```python
from build123d import *

# Parameters (mm, degrees)
F1_DEPTH    = 2500
F2_T        = 5
F2_T3_DEPTH = 2510
F4_DEPTH    = 2


# Not quite as in the source:
# - a shell that OpenCascade refuses in one call is made with other operations: the cavity is built on its own and cut out


with BuildPart() as f1:
    # F0 (on Top) → F1 (new body)
    with BuildSketch(Plane.XY):
        with BuildLine():
            Line((243.3531384634, 9.5), (16.4544826719, 140.5))
            ThreePointArc((16.4544826719, 140.5), (10.418948766, 139.705406887), (9.624355653, 133.6698729811))
            Line((9.624355653, 133.6698729811), (10.874355653, 131.5048094716))
            Line((10.874355653, 131.5048094716), (10.5801270189, 131.3349364905))
            Line((10.5801270189, 131.3349364905), (9.3301270189, 133.5))
            ThreePointArc((9.3301270189, 133.5), (3.7059047745, 135.8296291314), (0, 131))
            Line((0, 131), (0, -131))
            ThreePointArc((0, -131), (3.7059047745, -135.8296291314), (9.3301270189, -133.5))
            Line((9.3301270189, -133.5), (10.5801270189, -131.3349364905))
            Line((10.5801270189, -131.3349364905), (10.874355653, -131.5048094716))
            Line((10.874355653, -131.5048094716), (9.624355653, -133.6698729811))
            ThreePointArc((9.624355653, -133.6698729811), (10.418948766, -139.705406887), (16.4544826719, -140.5))
            Line((16.4544826719, -140.5), (243.3531384634, -9.5))
            ThreePointArc((243.3531384634, -9.5), (245.6827675949, -3.8757777556), (240.8531384634, -0.1698729811))
            Line((240.8531384634, -0.1698729811), (238.3531384634, -0.1698729811))
            Line((238.3531384634, -0.1698729811), (238.3531384634, 0.1698729811))
            Line((238.3531384634, 0.1698729811), (240.8531384634, 0.1698729811))
            ThreePointArc((240.8531384634, 0.1698729811), (245.6827675949, 3.8757777556), (243.3531384634, 9.5))
        make_face()
    extrude(amount=F1_DEPTH)

    # F2: shell of thickness 5, made by hand


with BuildPart() as f2_core1:
    # F2_t2: copy of F1
    add(f1.part)

    # the walls: a layer under each face that stays
    f2_faces = [f2_core1.faces().sort_by_distance(p)[0] for p in [
        (129.9038105677, 75, 1250),
        (10.249355653, 132.5873412263, 1250),
        (10.727241336, 131.4198729811, 1250),
        (9.9551270189, 132.4174682453, 1250),
        (0, 0, 1250),
        (9.9551270189, -132.4174682453, 1250),
        (10.727241336, -131.4198729811, 1250),
        (10.249355653, -132.5873412263, 1250),
        (129.9038105677, -75, 1250),
        (239.6031384634, -0.1698729811, 1250),
        (238.3531384634, 0, 1250),
        (239.6031384634, 0.1698729811, 1250),
    ]]
    thicken(f2_faces, amount=-F2_T, mode=Mode.SUBTRACT)

    # F2_s4 → F2_t3 (cut)
    with BuildSketch(Plane.XY.offset(-5)):
        Polygon((10.8060543828, 131.5231107418), (15.2044826719, 134.0048094716), (17.7044826719, 129.6746824527), (13.374355653, 127.1746824527), align=None)
        Polygon((10.5984282891, 131.4032377607), (13.0801270189, 127.0048094716), (8.75, 124.5048094716), (6.25, 128.8349364905), align=None)
        Polygon((10.5984282891, -131.4032377607), (6.25, -128.8349364905), (8.75, -124.5048094716), (13.0801270189, -127.0048094716), align=None)
        Polygon((10.8060543828, -131.5231107418), (13.374355653, -127.1746824527), (17.7044826719, -129.6746824527), (15.2044826719, -134.0048094716), align=None)
        Polygon((238.4031384634, -0.1198729811), (238.3531384634, -5.1698729811), (233.3531384634, -5.1698729811), (233.3531384634, -0.1698729811), align=None)
        Polygon((238.4031384634, 0.1198729811), (233.3531384634, 0.1698729811), (233.3531384634, 5.1698729811), (238.3531384634, 5.1698729811), align=None)
    extrude(amount=F2_T3_DEPTH, mode=Mode.SUBTRACT)


with BuildPart() as f1_1:
    add(f1.part)

    # what is left inside the walls is the cavity
    f2_cavity = [f2_core1.part.solids().sort_by_distance(p)[0] for p in [
        (5.05, 0, 1666.666667),
    ]]
    add(f2_cavity, mode=Mode.SUBTRACT)

    # F3 (on face) → F4 (join)
    with BuildSketch(Plane(origin=(0, 0, 0), x_dir=(1, 0, 0), z_dir=(0, 0, -1))):
        Polygon((8.75, 124.5048094716), (5, 131), (5, -131), (8.75, -124.5048094716), (17.7044826719, -129.6746824527), (13.9544826719, -136.1698729811), (240.8531384634, -5.1698729811), (233.3531384634, -5.1698729811), (233.3531384634, 5.1698729811), (240.8531384634, 5.1698729811), (13.9544826719, 136.1698729811), (17.7044826719, 129.6746824527), align=None)
    extrude(amount=-F4_DEPTH)


solid = f1_1.part
```
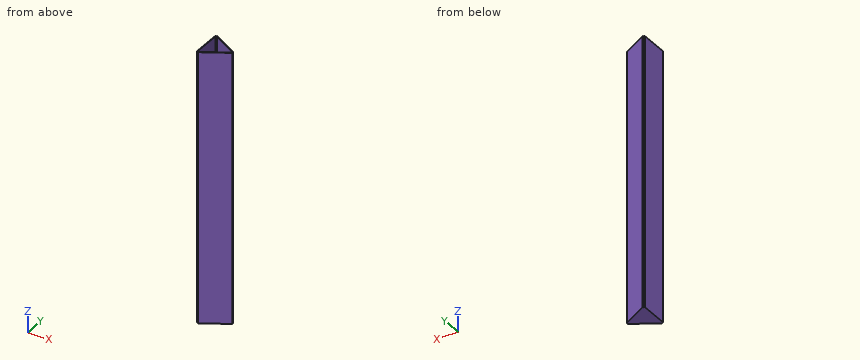
CAD build for the part. Positions are in the model's coordinates, mm. Round coordinates to 2 decimals unless told otherwise and drop trailing zeros. Order: outer loops, then holes, each group sorted by start corner. A loop starts at its lowest first (then second) coordinate and runs counter-clockwise, first axis right, second up. Notation, with made-up numbers: (-36.5, -3) -> (-20.5, -3) arc R23 cw to (-20.5, 7) -> close; hole circle Ø8 at (15.5, 58.25). An arc over 180 degrees is marked (long way). One line per question, with ' | ' between items.
Q1. Drop flat-ended pins along their axis: pin 1 (12 mm diameter, centred on y = -22, z = 2014, fed in from +X); pin 2 (2 mm diameter, centred on x = 239.5, z = 1022, fed in from -Y); pin 3 (12 mm diameter, centred on x = 170, z = 1380, fed in from -Y). Give the stop position or say it passes through.
Completed:
pin 1: stops at x = 232.09 | pin 2: stops at y = -12.3 | pin 3: stops at y = -55.31
Q2. Slice it at A-A (y = -54). Write the cut outline in (x, z), then the cut area to 3 significant figures.
Completed:
outline: (0, 0) -> (166.28, 0) -> (166.28, 2500) -> (156.28, 2500) -> (156.28, 2) -> (5, 2) -> (5, 2500) -> (0, 2500) -> close | area: 37,800 mm^2
Q3. Probe probe 1 along Z at (x, y) = (124, 19); probe 2 along Y at (x, z) = (137, 1020.5); probe 3 along Y at (x, z) = (131.5, 2093.5). List the from-to ranges inside material, lowest first.
Completed:
probe 1: z = 0 to 2 | probe 2: y = -70.9 to -65.13, 65.13 to 70.9 | probe 3: y = -74.08 to -68.3, 68.3 to 74.08
Q4. Slice it at B-B (x = 54). Write the cut outline in (y, z), then the cut area to 3 significant figures.
Completed:
outline: (-118.82, 0) -> (118.82, 0) -> (118.82, 2500) -> (113.05, 2500) -> (113.05, 2) -> (-113.05, 2) -> (-113.05, 2500) -> (-118.82, 2500) -> close | area: 29,300 mm^2
